For this review, take the finished solid that the model builds, in its own axes (mm). Face numbers are marked on the shaded views. A direction names the side the tool comes from. Round coordinates to 2 decimals unless told otherwise and drop trailing zeros. Order: outer loops, then holes, each group sorted by start corner. A loop starts at its lowest first (then second) coordinate and runs counter-clockwise, first axis right, second up. Notation, with made-up numbers: (60, 40) -> (84, 40) arc R6 cw to (84, 48) -> close; hole circle Ø7 at (-21, 43). An arc over 180 degrees is marked (long way). Use a Markdown table: item, result. Add a question column.
1) Clearance check with flat-ended pins moving along their axes: P1, Ø3, axis at y = -1, z = 3, coming from the -X side; P2, Ø1.5, axis at x = 9, z = 3, coming from the -Y side; P3, Ø5, axis at y = 0.5, z = 2.5, coming from the +X side. State where each tip first meets the part, or that it passes through.
2) Consider section A-A (y = 0). State the section outline as (x, z) points, plus the area to 3 significant figures.
3) Machinability: for the marked faces 4, 5 and 6, which of the approach directions +Z, -Z, +X, -X, +Y, -Y give a long, thin tool a straight path to every point of the face, cutting with its end or side? Answer none if there is none.
4) Draft analysis for pull direction X (two halves, no side actions). For the marked faces 1, 2 and 3, state which applies: pulls with the +X half, pulls with the -X half, needs draft (parallel to the pull), parting line crosses it, or undercut.
5) Wall thickness on line 1 along X through (y, z) = (-18, 6.75); line 2 along Z through (x, y) = (-14, -17); line 3 along X through (y, z) = (-4, 3): over which ranges is each line inside the solid? List them lowest first. Write a range as [from, to].
6) Consider section C-C (z = 9.25). State the section outline as (x, y) points.
7) Consider section B-B (x = -13). State the section outline as (y, z) points.
```python
from build123d import *

# Parameters (mm, degrees)
F0_R     = 1.5
F0_R_2   = 2.1
F1_DEPTH = 6
F2_R     = 3.88
F3_DEPTH = 26
F4_R     = 1.5
F5_DEPTH = 4
F6_SIZE  = 3.99999


# Not quite as in the source:
# - a fillet or chamfer is up to 0.001 mm smaller than in the source, because OpenCascade refuses the exact size


with BuildPart() as f1:
    # F0 (on Top) → F1 (new body)
    with BuildSketch(Plane.XY):
        with BuildLine():
            Line((4.5, 0), (4.5, 3.9686269666))
            ThreePointArc((4.5, 3.9686269666), (0, 6), (-4.5, 3.9686269666))
            Line((-4.5, 3.9686269666), (-4.5, 0))
            Line((-4.5, 0), (-4.5, -5.813701588))
            Line((-4.5, -5.813701588), (-15.143203234, -16.4569048219))
            ThreePointArc((-15.143203234, -16.4569048219), (-15.1189316865, -21.3823807428), (-10.1934557657, -21.4066522902))
            Line((-10.1934557657, -21.4066522902), (4.5, -7))
            Line((4.5, -7), (4.5, 0))
        make_face()
        with Locations((-12.6691633098, -18.9323580438)):
            Circle(F0_R, mode=Mode.SUBTRACT)
        Circle(F0_R_2, mode=Mode.SUBTRACT)
    extrude(amount=F1_DEPTH)

    # F2 (on face) → F3 (join)
    with BuildSketch(Plane(origin=(5.7049735344, -5.8185465008, 0), x_dir=(0.7140411723, 0.7001037097, 0), z_dir=(0.7001037097, -0.7140411723, 0))):
        with Locations((-11.9764822387, 6.39)):
            Circle(F2_R)
    extrude(amount=F3_DEPTH)

    # F4 (on face) → F5 (join)
    with BuildSketch(Plane.XY.offset(6)):
        with BuildLine():
            Line((-4.5, -5.813701588), (-15.143203234, -16.4569048219))
            ThreePointArc((-15.143203234, -16.4569048219), (-15.1189316865, -21.3823807428), (-10.1934557657, -21.4066522902))
            Line((-10.1934557657, -21.4066522902), (-5.6031765259, -16.9059713084))
            Line((-5.6031765259, -16.9059713084), (-0.0762481345, -11.4869237515))
            Line((-0.0762481345, -11.4869237515), (4.5, -7))
            Line((4.5, -7), (-4.5, -5.813701588))
        make_face()
        with Locations((-12.6691633098, -18.9323580438)):
            Circle(F4_R, mode=Mode.SUBTRACT)
    extrude(amount=F5_DEPTH)

    # F6 (size 4 in the source; OpenCascade refuses exactly that, so slightly less here)
    f6_edges = [f1.edges().sort_by_distance(p)[0] for p in [
        (0, -6.406851, 10),
    ]]
    chamfer(f6_edges, length=F6_SIZE)


solid = f1.part
```
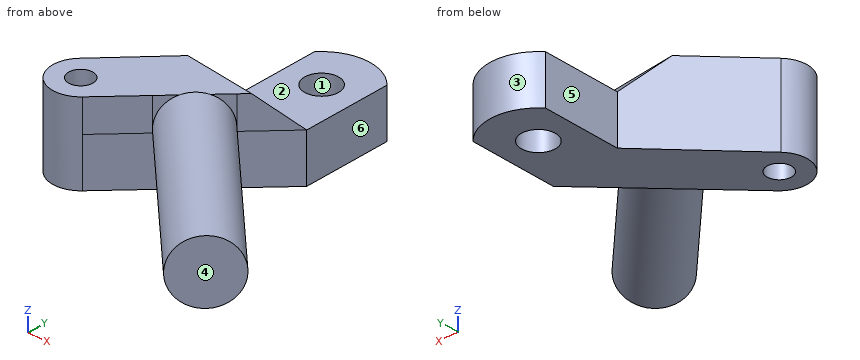
Results list:
| question | item | result |
|---|---|---|
| 1 | P1 | x = -4.5 |
| 1 | P2 | y = -30.6 |
| 1 | P3 | x = 4.5 |
| 2 | outline | (-4.5, 0) -> (-2.1, 0) -> (-2.1, 6) -> (-4.5, 6) -> close; (2.1, 0) -> (4.5, 0) -> (4.5, 6) -> (2.1, 6) -> close |
| 2 | area | 28.8 mm2 |
| 3 | face 4 | +Z, -Z, +X, -Y |
| 3 | face 5 | +Z, -Z, -X, +Y |
| 3 | face 6 | +Z, -Z, +X, +Y |
| 4 | face 1 | undercut |
| 4 | face 2 | needs draft |
| 4 | face 3 | parting line crosses it |
| 5 | line 1 | [-16.02, -13.84], [-11.49, -6.72], [-4.53, 6.29] |
| 5 | line 2 | [0, 10] |
| 5 | line 3 | [-4.5, 4.5] |
| 6 | outline | (-15.14, -16.46) arc R3.5 ccw to (-10.19, -21.41) -> (-4.72, -16.04) -> (13.48, -34.6) -> (17.23, -30.93) -> (-0.97, -12.37) -> (1.55, -9.89) -> (-7.4, -8.71) -> close; hole circle Ø3 at (-12.67, -18.93) |
| 7 | outline | (-22.39, 0) -> (-20.4, 0) -> (-20.4, 10) -> (-22.39, 10) -> close; (-17.47, 0) -> (-14.31, 0) -> (-14.31, 10) -> (-17.47, 10) -> close |
